For this review, take the finished solid that the model builds, in its own axes (mm). A direction names the side the tool comes from. Round coordinates to 2 decimals unless told otherwise and drop trailing zeros. Loops run counter-clockwise (first coordinate to the right, second up) from the corner with the lowest first, then second, coordinate; pieces in that order, holes last.
1) Mouldability with a two-part tool opening along X and no side actions: class faces 4 (the cylindrical face through (28.077, 113.099, 9.07)), 5 (the flat face through (52, 106, 0)), 6 (the cylindrical face through (42.3, 139.99, 9.07)) as pulls with the +X half, pulls with the -X half, needs draft (parallel to the pull), parting line crosses it, or undercut.
2) Take a section at A-A (x = 45). State the section outline as (y, z) points.
3) Take a section at D-D (y = 167). State the section outline as (x, z) points.
4) Wall thickness on L1, parallel to Y at x = 45.5, z = 0.5; L2, parallel to Y at x = 0, z = 3; L3, parallel to Z at x = 5.5, y = 13: over which ranges is each line inside the solid? List them lowest first.
5) Take a section at B-B (z = -4). State the section outline as (x, y) points.
6) Insertion check: pin 1 (16 mm diameter, centred on x = 50.5, y = 120.5, fed in from -Z); pin 2 (1.8 mm diameter, centred on y = 5.5, z = -0.5, fed in from -X); pin 3 (6 mm diameter, centred on x = 0, y = 0, fed in from -Z); pin 4 (11 mm diameter, centred on y = 159, z = 6.5, fed in from -X). Each pin has a flat end and moves straight along its axis. Give the tip position at first contact, or say it passes through.
7) Tool access review of faces 1 (the cylindrical face through (52.38, 187.14, 5.35)), 2 (the cylindrical face through (21.299, 77.786, 9.07)), 3 (the flat face through (15, 14, 9)): name each direction out of +Z, -Z, +X, -X, +Y, -Y from which nothing blocks a thin tool from reaching the whole face with its end or side.
8) Take a section at C-C (x = 22.5). State the section outline as (y, z) points.
Autodesk Inventor part; units mm, degrees
ref_plane "Arbeitsebene1" through (45, 112.9423, 0) normal (-1, 0, 0) x (0, 0, 1)
ref_plane "YZ Plane" through (0, 0, 0) normal (1, 0, 0) x (0, 1, 0)
ref_plane "XZ Plane" through (0, 0, 0) normal (0, 1, 0) x (-1, 0, 0)
sketch "Skizze1" plane through (0, 0, 0) normal (0, 0, 1) x (1, 0, 0)
  arc A0 (-1.5, 4.7697) -> (1.5, 4.7697) centre (0, 0) ccw
  circle A1 centre (0, 0) radius 12.5
  line L0 (-30.9429, 0) -> (77.0229, 0) construction
  circle A2 centre (0, 0) radius 15
  circle A3 centre (45, 112.9423) radius 16
  line L1 (61, 112.9423) -> (61, 172.9423)
  line L2 (29, 112.9423) -> (29, 172.9423)
  line L3 (45, 112.9423) -> (45, 188.9423) construction
  line L4 (45, 112.9423) -> (45, 128.9423) construction
  line L5 (29, 112.9423) -> (61, 112.9423) construction
  line L6 (-15, 0) -> (-15, 35)
  line L7 (15, 0) -> (15, 35)
  line L8 (-15, 35) -> (15, 35) construction
  circle A4 centre (0, 35) radius 15 construction
  line L9 (-12.8844, 42.6807) -> (29, 112.9423)
  arc A5 (-12.8844, 42.6807) -> (-15, 35) centre (0, 35) ccw
  line L10 (15, 35) -> (58.5544, 104.4407)
  arc A6 (58.5544, 104.4407) -> (61, 112.9423) centre (45, 112.9423) ccw
  line L11 (0, 35) -> (45, 112.9423) construction
  circle A7 centre (45, 172.9423) radius 16
  circle A8 centre (45, 172.9423) radius 9.5
  circle A9 centre (45, 112.9423) radius 9.5
  line L12 (-1.5, 6.4) -> (1.5, 6.4)
  line L13 (1.5, 6.4) -> (1.5, 4.7697)
  line L14 (-1.5, 4.7697) -> (-1.5, 6.4)
  line L15 (0, 0) -> (0, 5) construction
  line L16 (0, 5) -> (1.5, 5) construction
  circle A10 centre (45, 112.9423) radius 12.75 construction
  circle A11 centre (45, 172.9423) radius 12.75 construction
  line L17 (0, 0) -> (45, 172.9423) construction
  point P0 (22.5, 73.9711)
  point P1 (45, 142.9423)
  point P2 (-13, 0)
  point P3 (13, 0)
  point P4 (0, 6.4)
  point P5 (45, 125.6923)
  point P6 (33.9582, 106.5673)
  point P7 (56.0418, 106.5673)
  point P8 (45, 185.6923)
  point P9 (33.9582, 166.5673)
  point P10 (56.0418, 166.5673)
  dimension "d69" = 25.5
  dimension "ParallelHebel_Passflansch_HoleDia" = 25.5
  dimension "d0" = 10
  dimension "d1" = 25
  dimension "d4" = 30
  dimension "d36" = 0
  dimension "ParallelHebel_Gabelgelenk_OuterDia" = 32
  dimension "d38" = 60
  dimension "d39" = 35
  dimension "d40" = 90
  dimension "d41" = 60
  dimension "d42" = 45
  dimension "d43" = 19
  dimension "Nadellager_OuterDia" = 19
  dimension "d45" = 30
  dimension "d51" = 3
  dimension "d52" = 1.4
  dimension "d67" = 360
  dimension "d72" = 360
  dimension "Distanze_daVinciHead_Pivot" = 172.9423
extrude "Extrusion1" add sketch "Skizze1" against normal blind 10 contours A1
extrude "Extrusion2" add sketch "Skizze1" along normal blind 14 contours A1 | A2 | A2 L6 A5 L9 A3 L10 L7 | A3 | L2 A7 L1 A3 | A7
extrude "Extrusion4" cut sketch "Skizze1" along normal blind 4 contours A2 | A2 L6 A5 L9 A3 L10 L7 | L2 A7 L1 A3
fillet "Rundung1" radius 25 2 edges at (29, 112.9423, 9) (15, 35, 9)
hole "Bohrung2" at (45, 142.9423, 0) at (22.5, 73.9711, 0) direction (0, 0, 1) diameter 8 end through all
ref_plane "Arbeitsebene1" through (45, 112.9423, 0) normal (-1, 0, 0) x (0, 0, 1)
sketch "Skizze4" plane through (15, 0, 14) normal (1, 0, 0) x (0, 0, -1)
  line L0 (24, -12.5) -> (24, 12.5) construction
  line L1 (10, 41.0923) -> (10, 104.4407) construction
  line L2 (0, 41.0923) -> (0, 104.4407) construction
  line L3 (10, 112.9423) -> (10, 172.9423) construction
  line L4 (14, 156.9423) -> (14, 188.9423) construction
  point P0 (14, 0)
  dimension "ParallelMech_Distance_Step2Flat" = 14
  dimension "TrueLeverThickness" = 10
  dimension "ParallelMecha_BearingSide_Step" = 4
equation "\"NKX_10_RiadialPart_Dia\" = 19"
equation "\"Lager_Bohrung_Durchmesser\" = 19"
equation "\"Lager_Einbautiefe\" = 14"
properties part number "ParallelSystem_ProximalPart_Driven_v2.1_AxialNadellager" material "Edelstahl"
Response:
1. face 4: pulls with the -X half
1. face 5: needs draft
1. face 6: undercut
2. outline: (82.83, 4) - (96.94, 4) - (96.94, 0) - (103.44, 0) - (103.44, 14) - (82.83, 14) - close; (122.44, 0) - (128.94, 0) - (128.94, 4) - (138.94, 4) - (138.94, 14) - (122.44, 14) - close; (146.94, 4) - (156.94, 4) - (156.94, 0) - (163.44, 0) - (163.44, 14) - (146.94, 14) - close; (182.44, 0) - (188.94, 0) - (188.94, 14) - (182.44, 14) - close
3. outline: (29, 4) - (30.14, 4) - (30.14, 0) - (37.59, 0) - (37.59, 14) - (29, 14) - close; (52.41, 0) - (59.86, 0) - (59.86, 4) - (61, 4) - (61, 14) - (52.41, 14) - close
4. L1: y = 96.95 to 103.46, 122.43 to 128.93, 156.95 to 163.46, 182.43 to 188.93
4. L2: y = -12.5 to -5, 6.4 to 12.5
4. L3: z = 4 to 14
5. outline: circle Ø25 at (0, 0); hole (-1.5, 4.77) arc R5 ccw (long way) to (1.5, 4.77) - (1.5, 6.4) - (-1.5, 6.4) - close
6. pin 1: stops at z = 0
6. pin 2: stops at x = -11.62
6. pin 3: passes through
6. pin 4: stops at x = 29
7. face 1: -Z
7. face 2: +Z, -Z
7. face 3: +Z, -Z, +X, -Y
8. outline: (46.96, 4) - (69.97, 4) - (69.97, 14) - (46.96, 14) - close; (77.97, 4) - (102.04, 4) - (102.04, 14) - (77.97, 14) - close
